```python
from build123d import *

# Parameters (mm, degrees)
SKETCH1_R           = 16
BOSS_EXTRUDE1_DEPTH = 26.88
SKETCH4_R           = 9
BOSS_EXTRUDE2_DEPTH = 2
SKETCH5_R           = 9
BOSS_EXTRUDE3_DEPTH = 2
SKETCH6_R           = 7.5
CUT_EXTRUDE2_DEPTH  = 31.88
SKETCH7_R           = 1.615
CUT_EXTRUDE3_DEPTH  = 29.88


with BuildPart() as part:
    # Sketch1 → Boss-Extrude1 (new body)
    with BuildSketch(Plane.XY):
        Circle(SKETCH1_R)
    extrude(amount=BOSS_EXTRUDE1_DEPTH)

    # Sketch4 → Boss-Extrude2 (add)
    with BuildSketch(Plane.XY.offset(26.88)):
        Circle(SKETCH4_R)
    extrude(amount=BOSS_EXTRUDE2_DEPTH)

    # Sketch5 → Boss-Extrude3 (add)
    with BuildSketch(Plane(origin=(0, 0, 0), x_dir=(-1, 0, 0), z_dir=(0, 0, -1))):
        Circle(SKETCH5_R)
    extrude(amount=BOSS_EXTRUDE3_DEPTH)

    # Sketch6 → Cut-Extrude2 (cut, through all)
    with BuildSketch(Plane.XY.offset(28.88)):
        Circle(SKETCH6_R)
    extrude(amount=-CUT_EXTRUDE2_DEPTH, mode=Mode.SUBTRACT)

    # Sketch7 → Cut-Extrude3 (cut, through all)
    with BuildSketch(Plane.XY.offset(26.88)):
        with Locations((-8.485, 8.485)):
            Circle(SKETCH7_R)
        with Locations((8.485, 8.485)):
            Circle(SKETCH7_R)
        with Locations((8.485, -8.485)):
            Circle(SKETCH7_R)
        with Locations((-8.485, -8.485)):
            Circle(SKETCH7_R)
    extrude(amount=-CUT_EXTRUDE3_DEPTH, mode=Mode.SUBTRACT)


solid = part.part
```
Check sheet for the modelled part. Datum: model origin and axes. Units: mm. A direction names the side the tool comes from. Give positions to 0.01 mm unless a question says otherwise; leave off trailing zeros. Loops run counter-clockwise (first coordinate to the right, second up) from the corner with the lowest first, then second, coordinate; pieces in that order, holes last. Notation, with made-up numbers: (11.25, 81.25) - (23.25, 81.25) arc R8 ccw to (23.25, 87.25) - close; hole circle Ø11 at (40.25, 7). An arc over 180 degrees is marked (long way). One line per question, with ' | ' between items. Start each with the question number.
1. Draft check along Y on faces 1 (the cylindrical face through (-8.84, -10.06, 13.63)), 2 (the flat face through (7, -7, 26.88)), 3 (the cylindrical face through (1.172, 8.923, -0.986)). Enter one of: released by +Y, released by -Y, zero draft, split by the parting line, or undercut.
2. Set-up check for faces 4 (the cylindrical face through (-1.172, 8.923, 27.866)), 5 (the flat face through (2, 7.4, -2)), 6 (the flat face through (7, -7, 0)): record each of +Z, -Z, +X, -X, +Y, -Y from which the full face is reachable in a straight line by a thin tool's end or side.
3. Cross-section at C-C, the plane z = 4. Enter the section's corners in (x, y) (3 decimals).
4. Gauge pin test, flat ends, axial feed: pin 1 Ø2 at (y, z) = (2.5, 13.5) entering from -X; pin 2 Ø12 at (x, z) = (-11.5, 17.5) entering from +Y (3 decimals); pin 3 Ø3 at (x, y) = (-12.5, -7.5) entering from +Z; pin 4 Ø1.9 at (x, y) = (8.485, 8.485) entering from -Z. Record the tip position at first contact, or that the pin passes through.
5. Cross-section at D-D, the plane y = 14.5. Enter the section's corners in (x, z), plus the area to 3 significant figures.
6. Cross-section at A-A, the plane y = 0. Enter the section's corners in (x, z), plus the area to 3 significant figures.
7. Material ranges on line 1 along X through (y, z) = (-8, 3); line 2 along Y through (x, z) = (0, 21), recorded low to high. Write a range as [from, to].
Check result:
1) face 1: undercut | face 2: zero draft | face 3: split by the parting line
2) face 4: +Z | face 5: -Z, +X, -X, +Y, -Y | face 6: -Z
3) outline: circle Ø32 at (0, 0); hole circle Ø3.23 at (-8.485, -8.485); hole circle Ø3.23 at (-8.485, 8.485); hole circle Ø15 at (0, 0); hole circle Ø3.23 at (8.485, -8.485); hole circle Ø3.23 at (8.485, 8.485)
4) pin 1: stops at x = -15.93 | pin 2: stops at y = 15.025 | pin 3: stops at z = 26.88 | pin 4: passes through
5) outline: (-6.76, 0) - (6.76, 0) - (6.76, 26.88) - (-6.76, 26.88) - close | area: 364 mm2
6) outline: (-16, 0) - (-9, 0) - (-9, -2) - (-7.5, -2) - (-7.5, 28.88) - (-9, 28.88) - (-9, 26.88) - (-16, 26.88) - close; (7.5, -2) - (9, -2) - (9, 0) - (16, 0) - (16, 26.88) - (9, 26.88) - (9, 28.88) - (7.5, 28.88) - close | area: 469 mm2
7) line 1: x = [-13.86, -10.03], [-6.94, 6.94], [10.03, 13.86] | line 2: y = [-16, -7.5], [7.5, 16]
